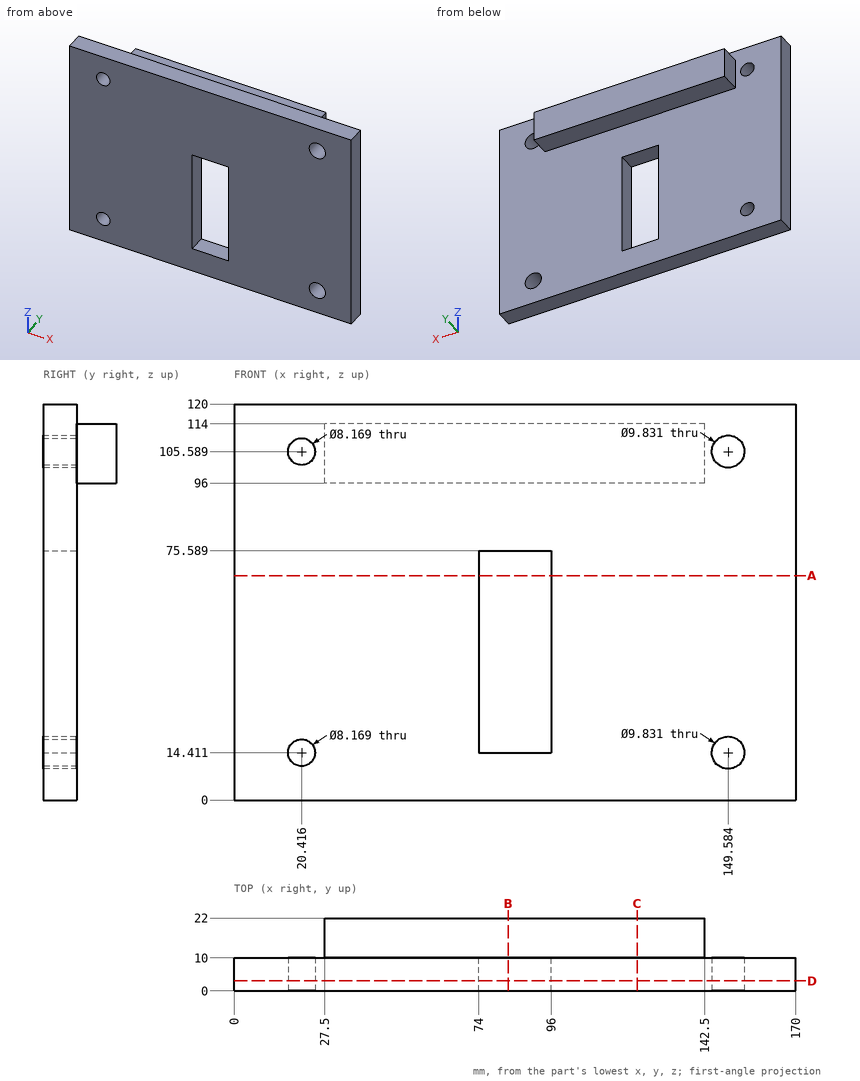
Can you work these out from the drawing? Everything is in mm from the part's minimum corner. Round coordinates to 2 decimals unless told otherwise and drop trailing zeros. Loops run counter-clockwise (first coordinate to the right, second up) from the corner with the lowest first, then second, coordinate; pieces in that order, holes last. Notation, with made-up numbers: (74, -13.5) - (89, -13.5) arc R22 cw to (89, 2.5) - close; hole circle Ø1 at (82, 69.5). An arc over 180 degrees is marked (long way). Answer in a Markdown table with one row per item. Add a question column.
Q1. I want a section at D-D on y = 3. List the corners of the cut face in (x, z) for me (1 decimal), and give its area (3 significant figures).
Q2. I want a section at A-A on z = 68. List the corners of the cut face in (x, y) for me.
Q3. I want a section at B-B on x = 83. List the corners of the cut face in (y, z) for me, and give its area (3 significant figures).
Q4. I want a section at C-C on x = 122. List the corners of the cut face in (y, z) for me, and give its area (3 significant figures).
Q5. For pin 1 Ø10 at (x, y) = (61, 19) entering from -Z; pin 2 Ø10.5 at (x, z) = (20.42, 14.41) entering from +Y; pin 3 Ø6 at (x, y) = (83.5, 13.5) entering from +Z, each with a flat end and sliding along its axis, tell me the tip position at first contact or that it passes through.
Q6. I need wall thicknesses on L1, parallel to X at y = 7, z = 23; L2, parallel to Z at x = 135.5, y = 12.25; L3, parallel to Y at x = 139.5, z = 31.5. Which ranges of each line are inside material? Lowest first, please.
A:
| question | item | result |
|---|---|---|
| 1 | outline | (0, 0) - (170, 0) - (170, 120) - (0, 120) - close; hole circle Ø8.2 at (20.4, 14.4); hole circle Ø8.2 at (20.4, 105.6); hole (74, 14.4) - (96, 14.4) - (96, 75.6) - (74, 75.6) - close; hole circle Ø9.8 at (149.6, 14.4); hole circle Ø9.8 at (149.6, 105.6) |
| 1 | area | 18,800 mm^2 |
| 2 | outline | (0, 0) - (74, 0) - (74, 10) - (0, 10) - close; (96, 0) - (170, 0) - (170, 10) - (96, 10) - close |
| 3 | outline | (0, 0) - (10, 0) - (10, 14.41) - (0, 14.41) - close; (0, 75.59) - (10, 75.59) - (10, 96) - (22, 96) - (22, 114) - (10, 114) - (10, 120) - (0, 120) - close |
| 3 | area | 804 mm^2 |
| 4 | outline | (0, 0) - (10, 0) - (10, 96) - (22, 96) - (22, 114) - (10, 114) - (10, 120) - (0, 120) - close |
| 4 | area | 1,420 mm^2 |
| 5 | pin 1 | z = 96 |
| 5 | pin 2 | y = 10 |
| 5 | pin 3 | z = 114 |
| 6 | L1 | 0 to 74, 96 to 170 |
| 6 | L2 | 96 to 114 |
| 6 | L3 | 0 to 10 |
